Input: part model. Units: mm. Frame: model coordinates. A direction names the side the tool comes from. Round coordinates to 2 decimals unless told otherwise and drop trailing zeros. Order: outer loops, then holes, each group sorted by start corner. A loop starts at its lowest first (then second) coordinate and runs counter-clockwise, first axis right, second up. Notation, with made-up numbers: (48.25, 75) -> (89.25, 75) arc R19 ccw to (89.25, 85) -> close; hole circle Ø6 at (3.5, 74.25). An arc over 180 degrees is marked (long way). Use a Markdown table: item, result.
from build123d import *

# Parameters (mm, degrees)
F1_DEPTH = 56


with BuildPart() as f1:
    # F0 (on Front) → F1 (new body)
    with BuildSketch(Plane.XZ):
        with BuildLine():
            Line((0, 35), (0, 5))
            Line((0, 5), (5.754496, 5))
            Line((5.754496, 5), (5.754496, 0))
            Line((5.754496, 0), (20.754496, 0))
            Line((20.754496, 0), (20.754496, 10))
            Line((20.754496, 10), (6.754496, 10))
            Line((6.754496, 10), (6.754496, 36.399462))
            ThreePointArc((6.754496, 36.399462), (3.448975, 35.353542), (0, 35))
        make_face()
        with BuildLine():
            Line((-21.245504, 0), (-6.245504, 0))
            Line((-6.245504, 0), (-6.245504, 5))
            Line((-6.245504, 5), (0, 5))
            Line((0, 5), (0, 35))
            ThreePointArc((0, 35), (-3.712349, 35.41029), (-7.245504, 36.621357))
            Line((-7.245504, 36.621357), (-7.245504, 10))
            Line((-7.245504, 10), (-21.245504, 10))
            Line((-21.245504, 10), (-21.245504, 0))
        make_face()
        with BuildLine():
            ThreePointArc((-7.245504, 36.621357), (-3.712349, 35.41029), (0, 35))
            ThreePointArc((0, 35), (3.448975, 35.353542), (6.754496, 36.399462))
            ThreePointArc((6.754496, 36.399462), (14.209617, 42.66797), (17, 52))
            ThreePointArc((17, 52), (-9.105669, 66.355723), (-7.245504, 36.621357))
        make_face()
        with BuildLine():
            ThreePointArc((11, 52), (7.778175, 44.221825), (0, 41))
            ThreePointArc((0, 41), (-7.778175, 59.778175), (11, 52))
        make_face(mode=Mode.SUBTRACT)
    extrude(amount=F1_DEPTH)


solid = f1.part
1) Set-up query: faces 4 (the face through (0, -28, 5)), 5 (the face through (-14, -28, 10)), 6 (the face through (6.754, -28, 23)), 7 (the face through (20.754, -28, 5)). Return all of +Z, -Z, +X, -X, +Y, -Y with unobstructed straight access to the full face (end or side cutting, diameter ignored); none if empty.
Answer key:
| item | result |
|---|---|
| face 4 | -Z, +Y, -Y |
| face 5 | -X, +Y, -Y |
| face 6 | +X, +Y, -Y |
| face 7 | +Z, -Z, +X, +Y, -Y |
2) Ray query, probe 1 along X at (y, z) = (-44, 52); probe 2 along Z at (x, y) = (-14, -47); probe 3 along Z at (x, y) = (-15.5, -7.5). Return the intervals inside material, ascending.
Answer key:
| item | result |
|---|---|
| probe 1 | x = -17 to -11, 11 to 17 |
| probe 2 | z = 0 to 10, 42.36 to 61.64 |
| probe 3 | z = 0 to 10, 45.02 to 58.98 |
3) Draft query along Z for faces 1 (the face through (-21.246, -28, 5)), 2 (the face through (13, -28, 0)), 3 (the face through (-7.246, -28, 23)). Return one class per face: released by +Z, released by -Z, zero draft, split by the parting line, or undercut.
Answer key:
| item | result |
|---|---|
| face 1 | zero draft |
| face 2 | released by -Z |
| face 3 | undercut |
4) Cut plane A-A on y = -28.5. Return loops of the section in (x, z).
Answer key:
| item | result |
|---|---|
| outline | (-21.25, 0) -> (-6.25, 0) -> (-6.25, 5) -> (5.75, 5) -> (5.75, 0) -> (20.75, 0) -> (20.75, 10) -> (6.75, 10) -> (6.75, 36.4) arc R17 ccw (long way) to (-7.25, 36.62) -> (-7.25, 10) -> (-21.25, 10) -> close; hole (0, 41) arc R11 ccw to (11, 52) arc R11 ccw (long way) to start |
5) Cut plane B-B on z = 42.5. Return loops of the section in (x, y).
Answer key:
| item | result |
|---|---|
| outline | (-14.1, -56) -> (-5.55, -56) -> (-5.55, 0) -> (-14.1, 0) -> close; (5.55, -56) -> (14.1, -56) -> (14.1, 0) -> (5.55, 0) -> close |
6) Cut plane D-D on z = 24.5. Return loops of the section in (x, y), and give its area (3 significant figures).
Answer key:
| item | result |
|---|---|
| outline | (-7.25, -56) -> (6.75, -56) -> (6.75, 0) -> (-7.25, 0) -> close |
| area | 784 mm^2 |
7) Contact query for flat-ended pins moving along their axis: P1, Ø8, axis at y = -29.5, z = 18.5, coming from the +X side; P2, Ø1.5, axis at x = -2, y = -16, coming from the +Z side; P3, Ø3.5, axis at x = -1.5, y = -16, coming from the -Z side. Output: stop coordinate, or through.
Answer key:
| item | result |
|---|---|
| P1 | stops at x = 6.75 |
| P2 | stops at z = 68.95 |
| P3 | stops at z = 5 |
8) Cut plane C-C on x = 16. Return loops of the section in (y, z), and give its area (3 significant figures).
Answer key:
| item | result |
|---|---|
| outline | (-56, 0) -> (0, 0) -> (0, 10) -> (-56, 10) -> close; (-56, 46.26) -> (0, 46.26) -> (0, 57.74) -> (-56, 57.74) -> close |
| area | 1,200 mm^2 |
